Part model, mm, in its own coordinate system. A direction names the side the tool comes from. Coordinates: 2 decimals unless noted, no trailing zeros. Loops run counter-clockwise (first coordinate to the right, second up) from the corner with the lowest first, then second, coordinate; pieces in that order, holes last. Notation, with made-up numbers: (54, 40) - (64, 40) arc R8 ccw to (64, 53) - close; hole circle Ø1 at (40.25, 3). An arc over 180 degrees is marked (long way). One line per question, with ' | ' between items. Start each with the question number.
from build123d import *

# Parameters (mm, degrees)
SKETCH1_W            = 275
SKETCH1_H            = 33
BOSS_EXTRUDE1_DEPTH  = 12
CUT_EXTRUDE1_REACH   = 141.005
SKETCH2_R            = 11
SKETCH2_R_2          = 2.5
SKETCH3_W            = 366
SKETCH3_H            = 117
BOSS_EXTRUDE2_DEPTH  = 12
CUT_EXTRUDE2_REACH   = 308.55
SKETCH4_R            = 2.5
CUT_EXTRUDE3_REACH   = 343.869
SKETCH5_W            = 14
SKETCH5_H            = 6
FILLET1_R            = 2
FILLET1_OF_MIRROR2_R = 2
CHAMFER1_SIZE        = 10
CUT_EXTRUDE4_REACH   = 343.869
SKETCH6_R            = 3
CUT_EXTRUDE6_REACH   = 343.869
SKETCH8_W            = 12
SKETCH8_H            = 42
CHAMFER2_SIZE        = 10


with BuildPart() as part:
    # Sketch1 → Boss-Extrude1 (new body)
    with BuildSketch(Plane.XY):
        Rectangle(SKETCH1_W, SKETCH1_H)
    extrude(amount=BOSS_EXTRUDE1_DEPTH)

    # Sketch2 → Cut-Extrude1 (cut, up to next)
    with BuildSketch(Plane.XY.offset(12), mode=Mode.PRIVATE) as cut_extrude1_sk1:
        with Locations((0, 1)):
            Circle(SKETCH2_R)
    cut_extrude1_tool1 = extrude(cut_extrude1_sk1.sketch, amount=-CUT_EXTRUDE1_REACH, mode=Mode.PRIVATE) & part.part
    # Sketch2 → Cut-Extrude1 (cut, up to next)
    with BuildSketch(Plane.XY.offset(12), mode=Mode.PRIVATE) as cut_extrude1_sk2:
        with Locations((-16.5, 1)):
            Circle(SKETCH2_R_2)
    cut_extrude1_tool2 = extrude(cut_extrude1_sk2.sketch, amount=-CUT_EXTRUDE1_REACH, mode=Mode.PRIVATE) & part.part
    # Sketch2 → Cut-Extrude1 (cut, up to next)
    with BuildSketch(Plane.XY.offset(12), mode=Mode.PRIVATE) as cut_extrude1_sk3:
        with Locations((16.5, 1)):
            Circle(SKETCH2_R_2)
    cut_extrude1_tool3 = extrude(cut_extrude1_sk3.sketch, amount=-CUT_EXTRUDE1_REACH, mode=Mode.PRIVATE) & part.part
    add(cut_extrude1_tool1.solids().sort_by_distance((0, 1, 12))[0], mode=Mode.SUBTRACT)
    add(cut_extrude1_tool2.solids().sort_by_distance((-16.5, 1, 12))[0], mode=Mode.SUBTRACT)
    add(cut_extrude1_tool3.solids().sort_by_distance((16.5, 1, 12))[0], mode=Mode.SUBTRACT)

    # Sketch3 → Boss-Extrude2 (add)
    with BuildSketch(Plane.XY.offset(12)):
        Polygon((-210, 16.5), (210, 16.5), (210, 46.5), (210, 269.5), (-210, 269.5), (-210, 46.5), align=None)
        with Locations((0, 105)):
            Rectangle(SKETCH3_W, SKETCH3_H, mode=Mode.SUBTRACT)
    extrude(amount=-BOSS_EXTRUDE2_DEPTH)

    # Sketch4 → Cut-Extrude2 (cut, up to next)
    with BuildSketch(Plane(origin=(0, 46.5, 0), x_dir=(1, 0, 0), z_dir=(0, 1, 0)), mode=Mode.PRIVATE) as cut_extrude2_sk1:
        with Locations(Location((-144, -6, 0), (0, 0, 270))):
            Circle(SKETCH4_R)
    cut_extrude2_tool1 = extrude(cut_extrude2_sk1.sketch, amount=-CUT_EXTRUDE2_REACH, mode=Mode.PRIVATE) & part.part
    # Sketch4 → Cut-Extrude2 (cut, up to next)
    with BuildSketch(Plane(origin=(0, 46.5, 0), x_dir=(1, 0, 0), z_dir=(0, 1, 0)), mode=Mode.PRIVATE) as cut_extrude2_sk2:
        with Locations(Location((-176, -6, 0), (0, 0, 270))):
            Circle(SKETCH4_R)
    cut_extrude2_tool2 = extrude(cut_extrude2_sk2.sketch, amount=-CUT_EXTRUDE2_REACH, mode=Mode.PRIVATE) & part.part
    cut_extrude2_1 = cut_extrude2_tool1.solids().sort_by_distance((-144, 46.5, 6))[0]
    add(cut_extrude2_1, mode=Mode.SUBTRACT)
    cut_extrude2_2 = cut_extrude2_tool2.solids().sort_by_distance((-176, 46.5, 6))[0]
    add(cut_extrude2_2, mode=Mode.SUBTRACT)
    cut_extrude2 = cut_extrude2_1 + cut_extrude2_2  # Cut-Extrude2 as one shape, for the pattern or mirror that repeats it

    # Mirror1: Cut-Extrude2 across plane
    add(cut_extrude2.mirror(Plane(origin=(0, 0, 0), x_dir=(0, 0, 1), z_dir=(1, 0, 0))), mode=Mode.SUBTRACT)

    # Sketch5 → Cut-Extrude3 (cut, up to next)
    with BuildSketch(Plane.XY.offset(12), mode=Mode.PRIVATE) as cut_extrude3_sk1:
        with Locations((-176, 43.5)):
            Rectangle(SKETCH5_W, SKETCH5_H)
    cut_extrude3_tool1 = extrude(cut_extrude3_sk1.sketch, amount=-CUT_EXTRUDE3_REACH, mode=Mode.PRIVATE) & part.part
    # Sketch5 → Cut-Extrude3 (cut, up to next)
    with BuildSketch(Plane.XY.offset(12), mode=Mode.PRIVATE) as cut_extrude3_sk2:
        with Locations((-144, 43.5)):
            Rectangle(SKETCH5_W, SKETCH5_H)
    cut_extrude3_tool2 = extrude(cut_extrude3_sk2.sketch, amount=-CUT_EXTRUDE3_REACH, mode=Mode.PRIVATE) & part.part
    cut_extrude3_1 = cut_extrude3_tool1.solids().sort_by_distance((-176, 43.5, 12))[0]
    add(cut_extrude3_1, mode=Mode.SUBTRACT)
    cut_extrude3_2 = cut_extrude3_tool2.solids().sort_by_distance((-144, 43.5, 12))[0]
    add(cut_extrude3_2, mode=Mode.SUBTRACT)
    cut_extrude3 = cut_extrude3_1 + cut_extrude3_2  # Cut-Extrude3 as one shape, for the pattern or mirror that repeats it

    # Fillet1
    fillet1_edges = [part.edges().sort_by_distance(p)[0] for p in [
        (-169, 40.5, 6),
        (-183, 40.5, 6),
        (-137, 40.5, 6),
        (-151, 40.5, 6),
    ]]
    fillet(fillet1_edges, radius=FILLET1_R)

    # Mirror2: Cut-Extrude3 across plane
    add(cut_extrude3.mirror(Plane(origin=(0, 0, 0), x_dir=(0, 0, 1), z_dir=(1, 0, 0))), mode=Mode.SUBTRACT)

    # Fillet1 of Mirror2
    fillet1_of_mirror2_edges = [part.edges().sort_by_distance(p)[0] for p in [
        (169, 40.5, 6),
        (183, 40.5, 6),
        (137, 40.5, 6),
        (151, 40.5, 6),
    ]]
    fillet(fillet1_of_mirror2_edges, radius=FILLET1_OF_MIRROR2_R)

    # Chamfer1
    chamfer1_edges = [part.edges().sort_by_distance(p)[0] for p in [
        (210, 16.5, 6),
        (-210, 16.5, 6),
    ]]
    chamfer(chamfer1_edges, length=CHAMFER1_SIZE)

    # Sketch6 → Cut-Extrude4 (cut, up to next)
    with BuildSketch(Plane.XY.offset(12), mode=Mode.PRIVATE) as cut_extrude4_sk1:
        with Locations((-194, 138.905602013)):
            Circle(SKETCH6_R)
    cut_extrude4_tool1 = extrude(cut_extrude4_sk1.sketch, amount=-CUT_EXTRUDE4_REACH, mode=Mode.PRIVATE) & part.part
    # Sketch6 → Cut-Extrude4 (cut, up to next)
    with BuildSketch(Plane.XY.offset(12), mode=Mode.PRIVATE) as cut_extrude4_sk2:
        with Locations((-194, 97.894768826)):
            Circle(SKETCH6_R)
    cut_extrude4_tool2 = extrude(cut_extrude4_sk2.sketch, amount=-CUT_EXTRUDE4_REACH, mode=Mode.PRIVATE) & part.part
    add(cut_extrude4_tool1.solids().sort_by_distance((-194, 138.905602, 12))[0], mode=Mode.SUBTRACT)
    add(cut_extrude4_tool2.solids().sort_by_distance((-194, 97.894769, 12))[0], mode=Mode.SUBTRACT)

    # Sketch8 → Cut-Extrude6 (cut, up to next)
    with BuildSketch(Plane.XY.offset(12), mode=Mode.PRIVATE) as cut_extrude6_sk1:
        with Locations((-194, 248.5)):
            Rectangle(SKETCH8_W, SKETCH8_H)
    cut_extrude6_tool1 = extrude(cut_extrude6_sk1.sketch, amount=-CUT_EXTRUDE6_REACH, mode=Mode.PRIVATE) & part.part
    # Sketch8 → Cut-Extrude6 (cut, up to next)
    with BuildSketch(Plane.XY.offset(12), mode=Mode.PRIVATE) as cut_extrude6_sk2:
        with Locations((194, 248.5)):
            Rectangle(SKETCH8_W, SKETCH8_H)
    cut_extrude6_tool2 = extrude(cut_extrude6_sk2.sketch, amount=-CUT_EXTRUDE6_REACH, mode=Mode.PRIVATE) & part.part
    add(cut_extrude6_tool1.solids().sort_by_distance((-194, 248.5, 12))[0], mode=Mode.SUBTRACT)
    add(cut_extrude6_tool2.solids().sort_by_distance((194, 248.5, 12))[0], mode=Mode.SUBTRACT)

    # Chamfer2
    chamfer2_edges = [part.edges().sort_by_distance(p)[0] for p in [
        (210, 269.5, 6),
        (-210, 269.5, 6),
    ]]
    chamfer(chamfer2_edges, length=CHAMFER2_SIZE - 0.0001)  # a hair under: the kernel refuses the full size


solid = part.part
1) Band-saw the part on A-A on y = 234.5. List the corners of the cut face in (x, z).
2) Pin check, flat tips, straight feed: pin 1 Ø4 at (y, z) = (18.5, 2) entering from -X; pin 2 Ø3 at (x, y) = (16.5, 1) entering from -Z. Stop position of each tip, or through.
3) Mould opens along X. For faces 1 (the flat face through (146.3, 40.5, 7.4)), 2 (the flat face through (-3, 192, 0)), 3 (the flat face through (205.1, 21.6, 6.1)), 4 (the flat face through (-137.5, 0, 6)) say: +X half, -X half, draft (parallel to the pull), parting line (faces both ways), or undercut.
4) Band-saw the part on C-C on y = 119. List the corners of the cut face in (x, z), then the cut area to 3 significant figures.
5) Wall check: line 1 along Y through (x, z) = (-194, 4.25); line 2 along Y through (x, z) = (-16.5, 9.75); line 3 along Y through (x, z) = (-103, 4). Give the ranges that are in metal, low to high. Write a range as [from, to].
6) Band-saw the part on B-B on x = 60. List the corners of the cut face in (y, z), then the cut area to 3 significant figures.
7) Tool access for faces 5 (the flat face through (-169, 16.5, 6)), 6 (the flat face through (137.5, 0, 6)), 7 (the flat face through (-146.3, 40.5, 7.4)), 8 (the flat face through (-194, 227.5, 6)): list every direction of +Z, -Z, +X, -X, +Y, -Y with a clear straight run to the whole face (end or side of a thin tool).
Values found:
1) outline: (-210, 0) - (-200, 0) - (-200, 12) - (-210, 12) - close; (-188, 0) - (188, 0) - (188, 12) - (-188, 12) - close; (200, 0) - (210, 0) - (210, 12) - (200, 12) - close
2) pin 1: x = -204 | pin 2: through
3) face 1: undercut | face 2: draft | face 3: +X half | face 4: -X half
4) outline: (-210, 0) - (-183, 0) - (-183, 12) - (-210, 12) - close; (183, 0) - (210, 0) - (210, 12) - (183, 12) - close | area: 648 mm²
5) line 1: [16.5, 94.89], [100.89, 135.91], [141.91, 227.5] | line 2: [-16.5, -1.5], [3.5, 46.5], [163.5, 269.5] | line 3: [-16.5, 46.5], [163.5, 269.5]
6) outline: (-16.5, 0) - (46.5, 0) - (46.5, 12) - (-16.5, 12) - close; (163.5, 0) - (269.5, 0) - (269.5, 12) - (163.5, 12) - close | area: 2,030 mm²
7) face 5: +Z, -Z, -X, -Y | face 6: +Z, -Z, +X, -Y | face 7: +Z, -Z | face 8: +Z, -Z, +Y
